Autodesk Inventor part; units mm, degrees
ref_plane "YZ Plane" through (0, 0, 0) normal (1, 0, 0) x (0, 1, 0)
ref_plane "XZ Plane" through (0, 0, 0) normal (0, 1, 0) x (-1, 0, 0)
ref_plane "XY Plane" through (0, 0, 0) normal (0, 0, 1) x (1, 0, 0)
ref_plane "Work Plane1" through (0, 0, 0) normal (0, 0, 1) x (1, 0, 0)
sketch "Sketch1" plane through (0, 0, 0) normal (0, 0, 1) x (1, 0, 0)
  line L0 (-83, -0.5) -> (-83, -81)
  line L1 (2, -82) -> (-93, -82)
  line L2 (-95, -2) -> (-95, -80)
  line L3 (-83, -81) -> (-96.6, -81)
  line L4 (-96.6, -81) -> (-96.6, 0)
  line L5 (-96.6, 0) -> (-83, 0)
  line L6 (-83, 0) -> (-83, -81)
  point P0 (0, 0)
  dimension "d0" = 1.6
extrude "Extrusion1" add sketch "Sketch1" against normal blind 2.4
sketch "Sketch2" plane through (0, 0, -2.4) normal (0, 0, -1) x (-1, 0, 0)
  line L0 (94, -9.5) -> (83, -9.5)
  line L1 (94, -57.961) -> (76.85, -57.961)
  line L2 (83, -81) -> (96.6, -81)
  line L3 (83, 0) -> (83, -81)
  line L4 (96.6, 0) -> (83, 0)
  line L5 (83, 0) -> (83, -9.1)
  line L6 (83, -9.1) -> (96.6, -9.1)
  line L7 (96.6, -9.1) -> (96.6, 0)
  point P0 (0, 0)
  dimension "d3" = 0.4
extrude "Extrusion2" add sketch "Sketch2" along normal blind 26.2
sketch "Sketch3" plane through (0, 0, -2.4) normal (0, 0, -1) x (-1, 0, 0)
  line L0 (96.6, -81) -> (96.6, -9.1)
  line L1 (83, -81) -> (96.6, -81)
  line L2 (96.6, -81) -> (96.6, -77)
  line L3 (96.6, -77) -> (83, -77)
  line L4 (83, -77) -> (83, -81)
  point P0 (0, 0)
  dimension "d6" = 4
extrude "Extrusion3" add sketch "Sketch3" along normal blind 5
sketch "Sketch4" plane through (-96.6, -81, 0) normal (-1, 0, 0) x (0, 0, 1)
  line L0 (-2.4, 71.9) -> (-2.4, 4)
  line L1 (-2.4, 71.9) -> (-10.4, 71.9)
  line L2 (-10.4, 71.9) -> (-10.4, 4)
  line L3 (-10.4, 4) -> (-2.4, 4)
  line L4 (-2.4, 4) -> (-2.4, 71.9)
  line L5 (-2.4, 4) -> (-7.4, 4)
  line L6 (-30, 1) -> (-30, 79)
  line L7 (-30, 71.9) -> (-13.7225, 71.9)
  line L8 (-13.7225, 71.9) -> (-13.7225, 4)
  line L9 (-13.7225, 4) -> (-30, 4)
  line L10 (-30, 4) -> (-30, 71.9)
  line L11 (-13.7225, 24.3406) -> (-13.7225, 32.8941)
  line L12 (-28.6, 71.9) -> (-30, 71.9)
  line L13 (-30, 71.9) -> (-30, 81)
  line L14 (-30, 81) -> (-28.6, 81)
  line L15 (-28.6, 81) -> (-28.6, 71.9)
  point P0 (0, 81)
  dimension "d9" = 8
extrude "Extrusion4" add sketch "Sketch4" against normal blind 1.6
sketch "Sketch5" plane through (-96.6, -81, 0) normal (-1, 0, 0) x (0, 0, 1)
  line L0 (-19.219, 23) -> (-0.5, 23)
  line L1 (-2, -1) -> (-28, -1)
  line L2 (-30, 81) -> (-30, 4)
  line L3 (0, 81) -> (0, 0)
  line L4 (0, 23) -> (-30, 23)
  line L5 (-30, 23) -> (-30, -1)
  line L6 (-30, -1) -> (0, -1)
  line L7 (0, -1) -> (0, 23)
  point P0 (-0.5, 23)
  point P1 (-28, -1)
extrude "Extrusion5" add sketch "Sketch5" against normal blind 1.6
sketch "Sketch6" plane through (-83, -81, -7.4) normal (0, -1, 0) x (1, 0, 0)
  circle A0 centre (-5.5, 3.4) radius 1.75
  circle A1 centre (-5.5, 3.4) radius 1.5
  point P0 (83, 7.4)
  dimension "d14" = 3
extrude "Extrusion6" add sketch "Sketch6" along normal blind 1.6 contours A1
sketch "Sketch7" plane through (0, 0, -28.6) normal (0, 0, -1) x (-1, 0, 0)
  circle A0 centre (90.5, -5.5) radius 1.75
  circle A1 centre (90.5, -5.5) radius 2
  point P0 (0, 0)
  dimension "d17" = 4
extrude "Extrusion7" cut sketch "Sketch7" against normal blind 12 contours A0 | A1
sketch "Sketch9" plane through (-96.6, 0, 0) normal (0, 1, 0) x (1, 0, 0)
  line L0 (3.1, 16) -> (9.1, 16)
  line L1 (9.1, 16) -> (9.1, 19)
  line L2 (9.1, 19) -> (3.1, 19)
  line L3 (3.1, 19) -> (3.1, 16)
  line L4 (0, 30) -> (1.6, 30)
  line L5 (4.1, 28.6) -> (4.1, 16.6)
  line L6 (8.1, 28.6) -> (8.1, 16.6)
  line L7 (6.1, 36) -> (6.1, -6)
  point P0 (96.6, 0)
  dimension "d23" = 3
  dimension "d24" = 6
  dimension "d25" = 11
  dimension "d26" = 3
extrude "Extrusion8" cut sketch "Sketch9" against normal through all
properties part number "Main"
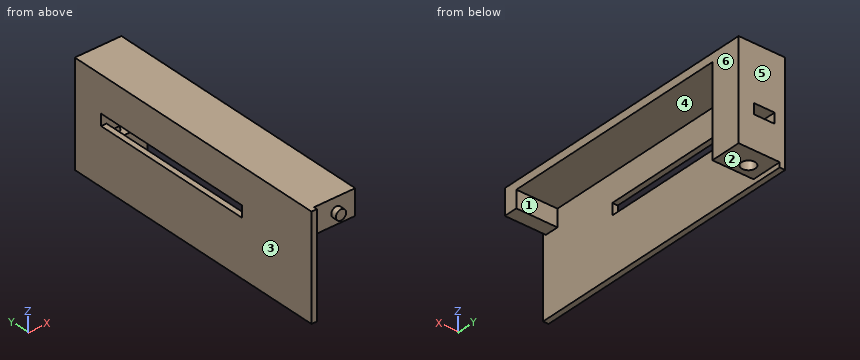
Part model, mm, in its own coordinate system. Face numbers are marked on the shaded views. A direction names the side the tool comes from. Round coordinates to 2 decimals unless told otherwise and drop trailing zeros. Loops run counter-clockwise (first coordinate to the right, second up) from the corner with the lowest first, then second, coordinate; pieces in that order, holes last.
Item 1: Drill centre lines: line 1 (Y direction, x = -86.5, z = -3); line 2 (Z direction, x = -95.75, y = -14); line 3 (Y direction, x = -90.5, z = -24.75). Where is each one in solid material? Low to high.
Item 2: 3-axis set-ups, long thin cutter, end or side, ignore diameter. For the marked faces 1, 2 and 3: which of +Z, -Z, +X, -X, +Y, -Y reach the whole face in a straight line?
Item 3: Cut at A-A, the plane z = -21.75. Give the cut face in (x, y), then the cut area to 3 significant figures.
Item 4: Drop flat-ended pins along their axis: P1, Ø1, axis at x = -88, y = -12.5, coming from the -Z side; P2, Ø2.5, axis at x = -89.5, y = -5.5, coming from the -Z side; P3, Ø3, axis at x = -87.5, z = -21, coming from the -Y side. Give the stop position or say it passes through.
Item 5: Mould opens along Y. For the marked faces 4, 5 and 6 say: +Y half, -Y half, draft (parallel to the pull), parting line (faces both ways), or undercut.
Item 6: Cut at C-C, the plane x = -90.75. Give the cut face in (y, z), then the cut area to 3 significant figures.
Item 7: Cut at D-D, the plane z = -4. Give the cut face in (x, y).
Item 8: Cut at B-B, the plane y = -10.5. Give the cut face in (x, z), then the cut area to 3 significant figures.
A:
1. line 1: y = -81 to -77, -9.1 to 0
1. line 2: z = -30 to -13.72, -10.4 to 0
1. line 3: y = -9.1 to -7.5, -3.5 to 0
2. face 1: -Z, +X
2. face 2: -Z, +X, +Y, -Y
2. face 3: +Z, -Z, -X, +Y, -Y
3. outline: (-96.6, -82) - (-95, -82) - (-95, -9.1) - (-83, -9.1) - (-83, 0) - (-96.6, 0) - close; hole circle Ø4 at (-90.5, -5.5)
3. area: 228 mm2
4. P1: stops at z = -2.4
4. P2: stops at z = -28.6
4. P3: stops at y = -9.1
5. face 4: undercut
5. face 5: +Y half
5. face 6: draft
6. outline: (-81, -7.4) - (-77, -7.4) - (-77, -2.4) - (-9.1, -2.4) - (-9.1, -16) - (0, -16) - (0, 0) - (-81, 0) - close; (-9.1, -28.6) - (-7.48, -28.6) - (-7.48, -19) - (-9.1, -19) - close; (-3.52, -28.6) - (0, -28.6) - (0, -19) - (-3.52, -19) - close
6. area: 387 mm2
7. outline: (-96.6, -82) - (-95, -82) - (-95, -81) - (-90, -81) - (-90, -82.6) - (-87, -82.6) - (-87, -81) - (-83, -81) - (-83, -77) - (-95, -77) - (-95, -9.1) - (-83, -9.1) - (-83, 0) - (-96.6, 0) - close
8. outline: (-96.6, -30) - (-95, -30) - (-95, -13.72) - (-96.6, -13.72) - close; (-96.6, -10.4) - (-95, -10.4) - (-95, -2.4) - (-83, -2.4) - (-83, 0) - (-96.6, 0) - close
8. area: 71.5 mm2
